Geometry: final body of the model. Coordinates: model frame, mm. Face numbers are marked on the shaded views. A direction names the side the tool comes from. Round coordinates to 2 decimals unless told otherwise and drop trailing zeros. Loops run counter-clockwise (first coordinate to the right, second up) from the corner with the lowest first, then second, coordinate; pieces in that order, holes last. Notation, with made-up numbers: (26.25, 30) - (54.25, 30) arc R22 cw to (54.25, 69) - close; hole circle Ø1 at (-0.75, 25.5). An arc over 180 degrees is marked (long way). Write item = value, one per line. Start each with the question number.
Item 1: Line query: line 1 (Y direction, x = -2.75, z = -2.75); line 2 (Y direction, x = 1, z = -1.75); line 3 (Y direction, x = 2.5, z = -0.5). Output: solid intervals per line, ascending. Write a range as from..to.
Item 2: Section A-A (y = 3.75). Return loops of the section in (x, z) (3 decimals).
Item 3: Draft query along Z for the marked faces 5, 6 and 7. Return one class per face: pulls with the +Z half, pulls with the -Z half, needs draft (parallel to the pull), parting line crosses it, or undercut.
Item 4: First-contact query: pin 1 (2.5 mm diameter, centred on x = 2, z = -1.5, fed in from -Y); pin 2 (2 mm diameter, centred on y = -6.5, z = 3, fed in from -X); pin 3 (0.7 mm diameter, centred on x = -1.5, y = -13, fed in from +Z). Flat tips, straight axial feed; report the tip coordinate or a pass-through.
Item 5: Access query for the marked faces 1, 2, 3 and 4. Directions: +Z, -Z, +X, -X, +Y, -Y. A direction counts if a zero-diameter tool reaches every point of the face in a straight line with its end or side. Return the directions, or none.
from build123d import *

# Parameters (mm, degrees)
SKETCH1_R           = 4.815
BOSS_EXTRUDE1_DEPTH = 2
SKETCH2_R           = 3.575
BOSS_EXTRUDE2_DEPTH = 7
SKETCH3_R           = 3.425
BOSS_EXTRUDE3_DEPTH = 6.85
SKETCH4_R           = 2.33
BOSS_EXTRUDE4_DEPTH = 5
SKETCH6_R           = 3
BOSS_EXTRUDE5_DEPTH = 0.67
BOSS_EXTRUDE6_START = 2.33
SKETCH7_R           = 3
SKETCH7_R_2         = 2.444387837
BOSS_EXTRUDE6_DEPTH = 2.33
SKETCH8_R           = 0.683030706
BOSS_EXTRUDE7_DEPTH = 2
SKETCH9_W           = 2.23373787
SKETCH9_H           = 6.792121548
CUT_EXTRUDE1_DEPTH  = 23.571638177
FILLET2_R           = 0.5
FILLET3_R           = 0.5


with BuildPart() as part:
    # Sketch1 → Boss-Extrude1 (new body)
    with BuildSketch(Plane(origin=(0, 0, 0), x_dir=(1, 0, 0), z_dir=(0, 1, 0))):
        with Locations(Location((0, 0, 0), (0, 0, 270))):
            Circle(SKETCH1_R)
    extrude(amount=-BOSS_EXTRUDE1_DEPTH)

    # Sketch2 → Boss-Extrude2 (add)
    with BuildSketch(Plane.XZ.offset(2)):
        with Locations(Location((0, 0, 0), (0, 0, 90))):
            Circle(SKETCH2_R)
    extrude(amount=BOSS_EXTRUDE2_DEPTH)

    # Sketch3 → Boss-Extrude3 (add)
    with BuildSketch(Plane(origin=(0, 0, 0), x_dir=(1, 0, 0), z_dir=(0, 1, 0))):
        with Locations(Location((0, 0, 0), (0, 0, 90))):
            Circle(SKETCH3_R)
    extrude(amount=BOSS_EXTRUDE3_DEPTH)

    # Sketch4 → Boss-Extrude4 (add)
    with BuildSketch(Plane(origin=(0, 6.85, 0), x_dir=(1, 0, 0), z_dir=(0, 1, 0))):
        with Locations(Location((0, 0, 0), (0, 0, 270))):
            Circle(SKETCH4_R)
    extrude(amount=BOSS_EXTRUDE4_DEPTH)

    # Sweep1: sweep along a curve in space
    with BuildLine() as sweep1_path:
        ThreePointArc((0, 6.85, 2.33), (1.6475588, 6.85, 1.6475588), (2.33, 6.85, 0))
        ThreePointArc((2.33, 6.85, 0), (1.6475588, 6.85, -1.6475588), (0, 6.85, -2.33))
        ThreePointArc((0, 6.85, -2.33), (-1.6475588, 6.85, -1.6475588), (-2.33, 6.85, 0))
        ThreePointArc((-2.33, 6.85, 0), (-1.6475588, 6.85, 1.6475588), (0, 6.85, 2.33))
    # Sketch5 → Sweep1 (sweep)
    with BuildSketch(Plane.XY):
        Polygon((-3.425, 6.85), (-2.33, 7.945), (-2.33, 6.85), align=None)
    sweep(path=sweep1_path.line)

    # Sketch6 → Boss-Extrude5 (add)
    with BuildSketch(Plane(origin=(0, 11.85, 0), x_dir=(1, 0, 0), z_dir=(0, 1, 0))):
        with Locations(Location((0, 0, 0), (0, 0, 270))):
            Circle(SKETCH6_R)
    extrude(amount=BOSS_EXTRUDE5_DEPTH)

    # Sketch7 → Boss-Extrude6 (add)
    with BuildSketch(Plane.XZ.offset(-11.85).offset(BOSS_EXTRUDE6_START)):
        with Locations(Location((0, 0, 0), (0, 0, 270))):
            Circle(SKETCH7_R)
        with Locations(Location((0, 0, 0), (0, 0, 270))):
            Circle(SKETCH7_R_2, mode=Mode.SUBTRACT)
    extrude(amount=-BOSS_EXTRUDE6_DEPTH)

    # Sketch8 → Boss-Extrude7 (add, symmetric)
    with BuildSketch(Plane(origin=(0, 0, 0), x_dir=(0, 0, -1), z_dir=(1, 0, 0))):
        with BuildLine():
            Line((-1.452989765, -9), (1.547010235, -9))
            Line((1.547010235, -9), (1.547010235, -12))
            Line((1.547010235, -12), (0.839903454, -12.707106781))
            Line((0.839903454, -12.707106781), (0.839903454, -13.707106781))
            Line((0.839903454, -13.707106781), (1.547010235, -14.414213562))
            Line((1.547010235, -14.414213562), (1.547010235, -14.914213562))
            ThreePointArc((1.547010235, -14.914213562), (0.047010235, -16.414213562), (-1.452989765, -14.914213562))
            Line((-1.452989765, -14.914213562), (-1.452989765, -14.414213562))
            Line((-1.452989765, -14.414213562), (-0.745882984, -13.707106781))
            Line((-0.745882984, -13.707106781), (-0.745882984, -12.707106781))
            Line((-0.745882984, -12.707106781), (-1.452989765, -12))
            Line((-1.452989765, -12), (-1.452989765, -9))
        make_face()
        with Locations((0.047010235, -14.914213562)):
            Circle(SKETCH8_R, mode=Mode.SUBTRACT)
    extrude(amount=BOSS_EXTRUDE7_DEPTH, both=True)

    # Sketch9 → Cut-Extrude1 (cut, through all)
    with BuildSketch(Plane.XZ.offset(9)):
        Rectangle(SKETCH9_W, SKETCH9_H)
    extrude(amount=CUT_EXTRUDE1_DEPTH, mode=Mode.SUBTRACT)

    # Fillet2
    fillet2_edges = [part.edges().sort_by_distance(p)[0] for p in [
        (0, 0, -4.815),
        (0, -2, -4.815),
    ]]
    fillet(fillet2_edges, radius=FILLET2_R)

    # Fillet3
    fillet3_edges = [part.edges().sort_by_distance(p)[0] for p in [
        (0, 12.52, -3),
    ]]
    fillet(fillet3_edges, radius=FILLET3_R)


solid = part.part
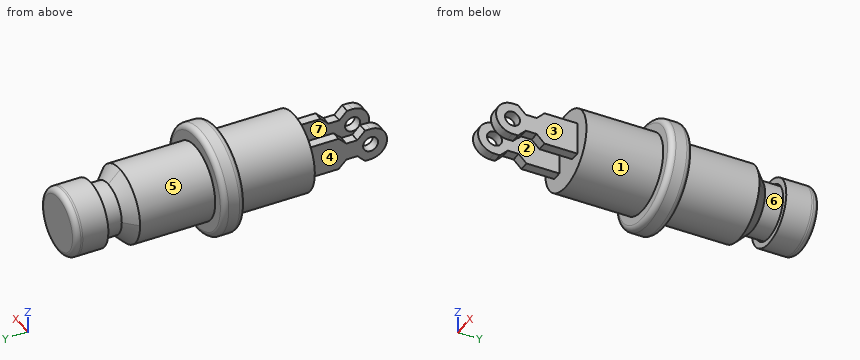
Taken from the geometry:
q1.line_1 = -2..0
q1.line_2 = -9..12.52
q1.line_3 = -9..7.73, 9.52..12.52
q2.outline = circle Ø6.85 at (0, 0)
q3.face_5 = parting line crosses it
q3.face_6 = undercut
q3.face_7 = needs draft
q4.pin_1 = -16.4
q4.pin_2 = -2.96
q4.pin_3 = 0.8
q5.face_1 = -Y
q5.face_2 = +Z, -Z, -Y
q5.face_3 = +Z, -Z, +X, -Y
q5.face_4 = +Z, -Z, -X, -Y
